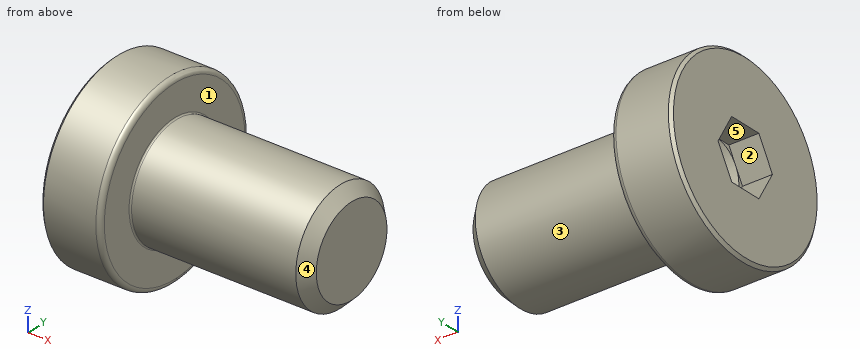
Autodesk Inventor part; units mm, degrees
ref_plane "screw_XY" through (0, 0, 0) normal (1, 0, 0) x (0, 0, -1)
ref_plane "screw_YZ" through (0, 0, 0) normal (0, 0, -1) x (0, 1, 0)
ref_plane "screw_ZX" through (0, 0, 0) normal (0, 1, 0) x (1, 0, 0)
sketch "Sketch_1" plane through (0, 0, 0) normal (0, 0, 1) x (1, 0, 0)
  line L0 (9.525, 0) -> (-3.226, 0)
  line L1 (-3.226, 0) -> (-3.226, 4.8476)
  line L2 (-3.226, 4.8476) -> (-3.0736, 5)
  line L3 (-3.0736, 5) -> (-0.254, 5)
  arc A0 (0, 4.746) -> (-0.254, 5) centre (-0.254, 4.746) ccw
  line L4 (0, 4.746) -> (0, 3.0762)
  arc A1 (0, 3.0762) -> (0.0762, 3) centre (0.0762, 3.0762) ccw
  line L5 (0.0762, 3) -> (8.9115, 3)
  line L6 (8.9115, 3) -> (9.525, 2.3865)
  line L7 (9.525, 2.3865) -> (9.525, 0)
  line L8 (9.525, 0) -> (-3.226, 0)
revolve "Revolution1" add sketch "Sketch_1" angle 360 about axis through (9.525, 0, 0) along (1, 0, 0)
thread "Thread1"
sketch "Sketch_3" plane through (-3.226, 0, 0) normal (1, 0, 0) x (0, 0, -1)
  line L0 (-1.5875, -0.9165) -> (0, -1.8331)
  line L1 (0, -1.8331) -> (1.5875, -0.9165)
  line L2 (1.5875, -0.9165) -> (1.5875, 0.9165)
  line L3 (1.5875, 0.9165) -> (0, 1.8331)
  line L4 (0, 1.8331) -> (-1.5875, 0.9165)
  line L5 (-1.5875, 0.9165) -> (-1.5875, -0.9165)
extrude "Extrusion1" cut sketch "Sketch_3" along normal blind 1.613
sketch "Sketch_4" plane through (0, 0, 0) normal (0, 0, 1) x (1, 0, 0)
  line L0 (-0.6965, 0) -> (-1.613, 0)
  line L1 (-1.613, 0) -> (-1.613, 1.5875)
  line L2 (-1.613, 1.5875) -> (-0.6965, 0)
  line L3 (-0.6965, 0) -> (-1.613, 0)
revolve "Revolution2" cut sketch "Sketch_4" angle 360 about axis through (-0.6965, 0, 0) along (1, 0, 0)
ref_plane "screw_XY" through (0, 0, 0) normal (1, 0, 0) x (0, 0, -1)
ref_plane "screw_YZ" through (0, 0, 0) normal (0, 0, -1) x (0, 1, 0)
ref_plane "screw_ZX" through (0, 0, 0) normal (0, 1, 0) x (1, 0, 0)
ref_plane "screw1_XY" through (9.525, 0, 0) normal (1, 0, 0) x (0, 0, -1)
ref_plane "screw1_YZ" through (9.525, 0, 0) normal (0, 0, -1) x (0, 1, 0)
ref_plane "screw1_ZX" through (9.525, 0, 0) normal (0, 1, 0) x (1, 0, 0)
ref_plane "screw2_XY" through (9.325, 0, 0) normal (1, 0, 0) x (0, 0, -1)
ref_plane "screw2_YZ" through (9.325, 0, 0) normal (0, 0, -1) x (0, 1, 0)
ref_plane "screw2_ZX" through (9.325, 0, 0) normal (0, 1, 0) x (1, 0, 0)
ref_plane "to_tnut_XY" through (0.29, 0, 0) normal (1, 0, 0) x (0, 0, -1)
ref_plane "to_tnut_YZ" through (0.29, 0, 0) normal (0, 0, -1) x (0, 1, 0)
ref_plane "to_tnut_ZX" through (0.29, 0, 0) normal (0, 1, 0) x (1, 0, 0)
properties part number "25-2750-6"
Work out the finished part from the listing and answer in its coordinate system (mm). Face numbers are marked on the shaded views. A direction names the side the tool comes from. Give positions to 0.01 mm unless a question says otherwise; leave off trailing zeros. Order: outer loops, then holes, each group sorted by start corner. A loop starts at its lowest first (then second) coordinate and runs counter-clockwise, first axis right, second up. Notation, with made-up numbers: (69, -39) - (73, -39) arc R28 cw to (73, -21) - close; hole circle Ø5 at (-34, -21). An arc over 180 degrees is marked (long way). One line per item, written item: value. Start each with the question number.
1. Section A-A, the plane x = 5.75 is taken. Write down the section's boundary in (y, z), then the cut area to 3 significant figures.
2. For a pull along Y with two mould halves and no side action, classify the marked faces 1, 2 and 3 as released by +Y, released by -Y, zero draft, split by the parting line, or undercut.
3. Consider line 1 (X direction, y = 0.25, z = -3.5); line 2 (Z direction, x = 2.75, y = 0); line 3 (Z direction, x = -2, y = -1.75). Determine where each line is inside the solid, lowest interval first.
4. Each of these flat-tipped pins is pushed along its axis until it touches: pin 1 Ø4 at (x, z) = (4, 3.5) entering from +Y; pin 2 Ø3 at (x, y) = (4.5, 1) entering from +Z; pin 3 Ø0.6 at (y, z) = (-0.5, 1.5) entering from -X; pin 4 Ø0.6 at (y, z) = (0.5, -1) entering from -X. Where does it stop, or does it pass through?
5. Which of the six approach directions +Z, -Z, +X, -X, +Y, -Y give full straight-line access (tool end or side, diameter ignored) to the marked faces 4 and 5?
Filled sheet:
1. outline: circle Ø6 at (0, 0)
1. area: 28.3 mm²
2. face 1: zero draft
2. face 2: undercut
2. face 3: split by the parting line
3. line 1: -3.23 to 0
3. line 2: -3 to 3
3. line 3: -4.68 to -0.14, 0.14 to 4.68
4. pin 1: y = 2.6
4. pin 2: z = 3
4. pin 3: x = -3.23
4. pin 4: x = -1.52
5. face 4: +X
5. face 5: -X
